from build123d import *

# Parameters (mm, degrees)
SKETCH1_W           = 40
SKETCH1_H           = 40
BOSS_EXTRUDE1_DEPTH = 5
FILLET1_R           = 3


with BuildPart() as part:
    # Sketch1 → Boss-Extrude1 (new body, symmetric)
    with BuildSketch(Plane.XY):
        with Locations((-20, 20)):
            Rectangle(SKETCH1_W, SKETCH1_H)
    extrude(amount=BOSS_EXTRUDE1_DEPTH, both=True)

    # Fillet1
    fillet1_edges = [part.edges().sort_by_distance(p)[0] for p in [
        (-40, 20, 5),
        (-20, 0, 5),
        (0, 20, 5),
        (0, 0, 0),
        (-40, 0, 0),
        (-40, 40, 0),
        (0, 40, 0),
        (-20, 40, 5),
    ]]
    fillet(fillet1_edges, radius=FILLET1_R)


solid = part.part
Can you work these out from the model? Positions are in its coordinate system, mm. Coordinates: 2 decimals unless noted, no trailing zeros. Write each loop counter-clockwise with the first axis right and the second up, starting at its lowest first coordinate (ties: lowest second). Pieces come first, ordered by that corner, then holes. Notation, with made-up numbers: (37.5, 33) - (89.5, 33) arc R27 ccw to (89.5, 68) - close; hole circle Ø2 at (-8.75, 52.25). An arc over 180 degrees is marked (long way). Return JSON: item names as keys, results as strings. Group by question number.
Item 1: Please list where these lines run through material, in increasing order: probe 1 along Y at (x, z) = (-19.5, 4.75); probe 2 along X at (y, z) = (29, 3.75); probe 3 along Y at (x, z) = (-24.5, 2.75).
Item 2: If we section it at A-A (x = -2.5): Write out the boundary of the cut face in (y, z), then the cut area to 3 significant figures.
Item 3: If we section it at B-B (z = 3.5): Write out the boundary of the cut face in (x, y).
Return value:
{
 "1": {"probe 1": "y = 1.8 to 38.2", "probe 2": "x = -39.44 to -0.56", "probe 3": "y = 0.1 to 39.9"},
 "2": {"outline": "(0.04, -5) - (39.96, -5) - (39.96, 2) arc R2.96 ccw to (37, 4.96) - (3, 4.96) arc R2.96 ccw to (0.04, 2) - close", "area": "394 mm^2"},
 "3": {"outline": "(-39.6, 3) arc R2.6 ccw to (-37, 0.4) - (-3, 0.4) arc R2.6 ccw to (-0.4, 3) - (-0.4, 37) arc R2.6 ccw to (-3, 39.6) - (-37, 39.6) arc R2.6 ccw to (-39.6, 37) - close"}
}
